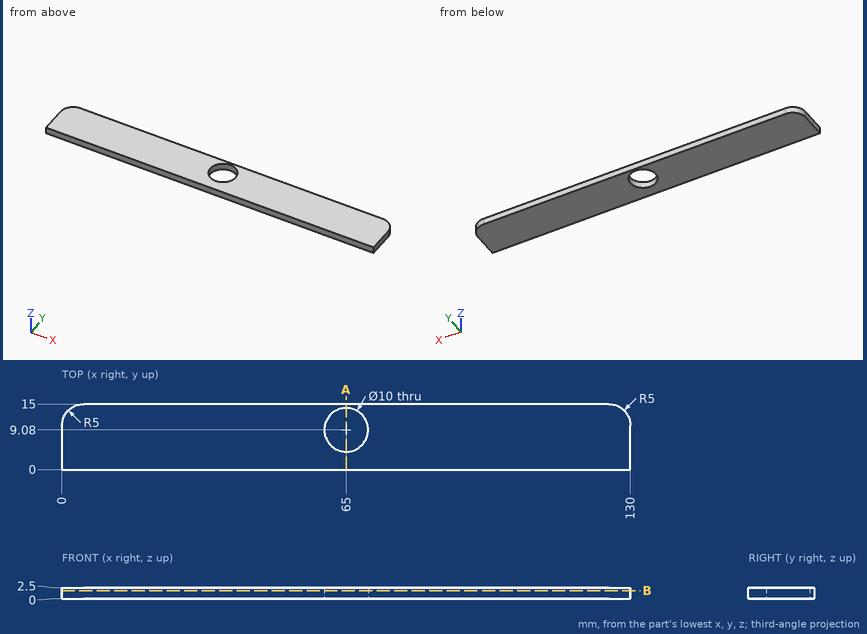
Input: dimensioned drawing with shaded views. Units: mm. Origin: part minimum x, y, z. Coordinates: 2 decimals unless noted, no trailing zeros. Loops run counter-clockwise (first coordinate to the right, second up) from the corner with the lowest first, then second, coordinate; pieces in that order, holes last. Notation, with made-up numbers: M -8,9 L 7,9 A19 ccw 7,43 Z; hole C 88,16 d2. An arc over 180 degrees is marked long. Use a Markdown table: item, result. Add a question column.
1) Section A-A, the plane x = 65. Return the cut outline in (y, z).
2) Pin query (flat end, axial travel): P1, Ø2, axis at x = 62, y = 4.5, coming from the -Z side. Return the tip coordinate at first contact, or that it passes through.
3) Section B-B, the plane z = 1.8. Return the cut outline in (x, y).
4) Line query: L1, parallel to X at y = 9.25, z = 1.5; L2, parallel to Y at x = 65, z = 1.3; L3, parallel to X at y = 6.5, z = 0.65. Output: solid intervals per line, ascending. Write a range as from..to.
Answer below:
| question | item | result |
|---|---|---|
| 1 | outline | M 0,0 L 4.08,0 L 4.08,2.5 L 0,2.5 Z; M 14.08,0 L 15,0 L 15,2.5 L 14.08,2.5 Z |
| 2 | P1 | z = 0 |
| 3 | outline | M 0,0 L 130,0 L 130,10 A5 ccw 125,15 L 5,15 A5 ccw 0,10 Z; hole C 65,9.08 d10 |
| 4 | L1 | 0..60, 70..130 |
| 4 | L2 | 0..4.08, 14.08..15 |
| 4 | L3 | 0..60.72, 69.28..130 |
